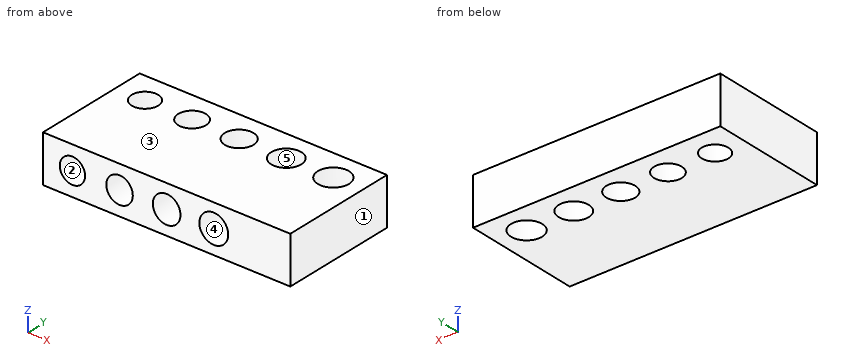
from build123d import *

# Parameters (mm, degrees)
SKETCH_1_W          = 42
SKETCH_1_H          = 20
EXTRUDE_1_DEPTH     = 8
SKETCH_2_R          = 2.25
SKETCH_2_R_2        = 2.35
SKETCH_2_R_3        = 2.45
SKETCH_2_R_4        = 2.55
SKETCH_2_R_5        = 2.65
CUT_EXTRUDE_1_DEPTH = 9
SKETCH_3_R          = 2.15
SKETCH_3_R_2        = 2.25
SKETCH_3_R_3        = 2.35
SKETCH_3_R_4        = 2.45
CUT_EXTRUDE_2_DEPTH = 10


with BuildPart() as part:
    # ｽｹｯﾁ1 → ﾎﾞｽ - 押し出し1 (new body)
    with BuildSketch(Plane.XY):
        Rectangle(SKETCH_1_W, SKETCH_1_H)
    extrude(amount=EXTRUDE_1_DEPTH)

    # ｽｹｯﾁ2 → ｶｯﾄ - 押し出し1 (cut, through all)
    with BuildSketch(Plane.XY.offset(8)):
        with Locations((-16, 5)):
            Circle(SKETCH_2_R)
        with Locations((-8, 5)):
            Circle(SKETCH_2_R_2)
        with Locations((0, 5)):
            Circle(SKETCH_2_R_3)
        with Locations((8, 5)):
            Circle(SKETCH_2_R_4)
        with Locations((16, 5)):
            Circle(SKETCH_2_R_5)
    extrude(amount=-CUT_EXTRUDE_1_DEPTH, mode=Mode.SUBTRACT)

    # ｽｹｯﾁ3 → ｶｯﾄ - 押し出し2 (cut)
    with BuildSketch(Plane.XZ.offset(10)):
        with Locations((-16, 4)):
            Circle(SKETCH_3_R)
        with Locations((-8, 4)):
            Circle(SKETCH_3_R_2)
        with Locations((0, 4)):
            Circle(SKETCH_3_R_3)
        with Locations((8, 4)):
            Circle(SKETCH_3_R_4)
    extrude(amount=-CUT_EXTRUDE_2_DEPTH, mode=Mode.SUBTRACT)


solid = part.part
Could you check a few things on this model? Use its own coordinates, in mm. Face numbers are marked on the shaded views. A direction names the side the tool comes from. Round coordinates to 2 decimals unless told otherwise and drop trailing zeros. Order: outer loops, then holes, each group sorted by start corner. A loop starts at its lowest first (then second) coordinate and runs counter-clockwise, first axis right, second up.
(1) Which directions (+Z, -Z, +X, -X, +Y, -Y) give clear straight access to the entire face, cutting with the end or side of a thin tool? Please do the marked faces 4 and 5.
Response values:
face 4: -Y
face 5: +Z, -Z
(2) Please list where these lines run through material, in increasing order: line 1 along Y through (x, z) = (-16, 5); line 2 along Y through (x, z) = (-8, 3.5); line 3 along Z through (x, y) = (8, -4).
Response values:
line 1: y = 0 to 2.75, 7.25 to 10
line 2: y = 0 to 2.65, 7.35 to 10
line 3: z = 0 to 1.55, 6.45 to 8
(3) Imagine slicing it at C-C (y = -1.25). Write out the boundary of the cut face in (x, z), plus the area to 3 significant figures.
Response values:
outline: (-21, 0) - (21, 0) - (21, 8) - (-21, 8) - close; hole circle Ø4.3 at (-16, 4); hole circle Ø4.5 at (-8, 4); hole circle Ø4.7 at (0, 4); hole circle Ø4.9 at (8, 4)
area: 269 mm2
(4) If we mould it in two halves opening along X, with no side actions, what happens to the marked faces 1, 2 and 3? For each: released by +X, released by -X, zero draft, split by the parting line, or undercut.
Response values:
face 1: released by +X
face 2: undercut
face 3: zero draft
(5) I'm going to push flat-ended pins straight in: pin 1 (1.4 mm diameter, centred on x = 0.5, z = 4, fed in from -Y); pin 2 (2.5 mm diameter, centred on x = -16, y = 5, fed in from -Z); pin 3 (6 mm diameter, centred on x = -11.5, y = -6, fed in from -Z). Where does each tip first touch, or does it pass through?
Response values:
pin 1: stops at y = 0
pin 2: passes through
pin 3: stops at z = 0
(6) Imagine slicing it at B-B (y = 5). Write out the boundary of the cut face in (x, z).
Response values:
outline: (-21, 0) - (-18.25, 0) - (-18.25, 8) - (-21, 8) - close; (-13.75, 0) - (-10.35, 0) - (-10.35, 8) - (-13.75, 8) - close; (-5.65, 0) - (-2.45, 0) - (-2.45, 8) - (-5.65, 8) - close; (2.45, 0) - (5.45, 0) - (5.45, 8) - (2.45, 8) - close; (10.55, 0) - (13.35, 0) - (13.35, 8) - (10.55, 8) - close; (18.65, 0) - (21, 0) - (21, 8) - (18.65, 8) - close
(7) Imagine slicing it at A-A (x = 8). Write out the boundary of the cut face in (y, z), plus the area to 3 significant figures.
Response values:
outline: (-10, 0) - (2.45, 0) - (2.45, 8) - (-10, 8) - (-10, 6.45) - (0, 6.45) - (0, 1.55) - (-10, 1.55) - close; (7.55, 0) - (10, 0) - (10, 8) - (7.55, 8) - close
area: 70.2 mm2
(8) Imagine slicing it at D-D (z = 4). Write out the boundary of the cut face in (x, y).
Response values:
outline: (-21, -10) - (-18.15, -10) - (-18.15, 0) - (-13.85, 0) - (-13.85, -10) - (-10.25, -10) - (-10.25, 0) - (-5.75, 0) - (-5.75, -10) - (-2.35, -10) - (-2.35, 0) - (2.35, 0) - (2.35, -10) - (5.55, -10) - (5.55, 0) - (10.45, 0) - (10.45, -10) - (21, -10) - (21, 10) - (-21, 10) - close; hole circle Ø4.5 at (-16, 5); hole circle Ø4.7 at (-8, 5); hole circle Ø4.9 at (0, 5); hole circle Ø5.1 at (8, 5); hole circle Ø5.3 at (16, 5)
